Work out the finished part from the listing and answer in its coordinate system (mm). Face numbers are marked on the shaded views. A direction names the side the tool comes from. Coordinates: 2 decimals unless noted, no trailing zeros. Write each loop counter-clockwise with the first axis right and the second up, starting at its lowest first coordinate (ties: lowest second). Pieces come first, ordered by that corner, then holes. Notation, with made-up numbers: (-34.5, 5) - (-6.5, 5) arc R16 cw to (-6.5, 29) - close; hole circle Ø2 at (18, -18). An arc over 180 degrees is marked (long way). Answer as a JSON object with one key per item and string values. Group by question number.
from build123d import *

# Parameters (mm, degrees)
SKETCH1_W           = 60
SKETCH1_H           = 30
SKETCH1_R           = 2.3
BOSS_EXTRUDE1_DEPTH = 5
SKETCH3_W           = 5
SKETCH3_H           = 5
BOSS_EXTRUDE2_DEPTH = 35
SKETCH5_W           = 5
SKETCH5_H           = 5
SKETCH5_R           = 1.875
BOSS_EXTRUDE3_DEPTH = 2.5
SKETCH6_W           = 5
SKETCH6_H           = 30
BOSS_EXTRUDE4_DEPTH = 15
CUT_EXTRUDE1_REACH  = 64.048


with BuildPart() as part:
    # Sketch1 → Boss-Extrude1 (new body)
    with BuildSketch(Plane.XY):
        Rectangle(SKETCH1_W, SKETCH1_H)
        with Locations((-13.800714267, 9.000714267)):
            Circle(SKETCH1_R, mode=Mode.SUBTRACT)
        with Locations((5.999285733, 9.000714267)):
            Circle(SKETCH1_R, mode=Mode.SUBTRACT)
        with Locations((20, -5)):
            Circle(SKETCH1_R, mode=Mode.SUBTRACT)
    extrude(amount=BOSS_EXTRUDE1_DEPTH)

    # Sketch3 → Boss-Extrude2 (add)
    with BuildSketch(Plane.XY.offset(5)):
        with Locations((27.5, 12.5)):
            Rectangle(SKETCH3_W, SKETCH3_H)
        with Locations((-27.5, -12.5)):
            Rectangle(SKETCH3_W, SKETCH3_H)
    extrude(amount=BOSS_EXTRUDE2_DEPTH)

    # Sketch5 → Boss-Extrude3 (add)
    # profile 1 of 2: a face of its own
    with BuildSketch(Plane.XY.offset(40)):
        with Locations((-27.5, -7.5)):
            Rectangle(SKETCH5_W, SKETCH5_H)
        with Locations((-27.5, -7.5)):
            Circle(SKETCH5_R, mode=Mode.SUBTRACT)
    # profile 2 of 2: a face of its own
    with BuildSketch(Plane.XY.offset(40)):
        with Locations((27.5, 7.5)):
            Rectangle(SKETCH5_W, SKETCH5_H)
        with Locations((27.5, 7.5)):
            Circle(SKETCH5_R, mode=Mode.SUBTRACT)
    extrude(amount=-BOSS_EXTRUDE3_DEPTH)

    # Sketch6 → Boss-Extrude4 (add)
    with BuildSketch(Plane.ZY.offset(30)):
        with Locations((2.5, 0)):
            Rectangle(SKETCH6_W, SKETCH6_H)
    extrude(amount=BOSS_EXTRUDE4_DEPTH)

    # Sketch7 → Cut-Extrude1 (cut, up to next)
    with BuildSketch(Plane(origin=(0, 0, 0), x_dir=(-1, 0, 0), z_dir=(0, 0, -1)), mode=Mode.PRIVATE) as cut_extrude1_sk1:
        with BuildLine():
            Line((23.394171206, 9.42), (39.386735103, 9.42))
            ThreePointArc((39.386735103, 9.42), (43.815453154, -0.09), (39.386735103, -9.6))
            Line((39.386735103, -9.6), (23.394171206, -9.6))
            ThreePointArc((23.394171206, -9.6), (18.965453154, -0.09), (23.394171206, 9.42))
        make_face()
    cut_extrude1_tool1 = extrude(cut_extrude1_sk1.sketch, amount=-CUT_EXTRUDE1_REACH, mode=Mode.PRIVATE) & part.part
    add(cut_extrude1_tool1.solids().sort_by_distance((-31.390453, -0.09, 0))[0], mode=Mode.SUBTRACT)


solid = part.part
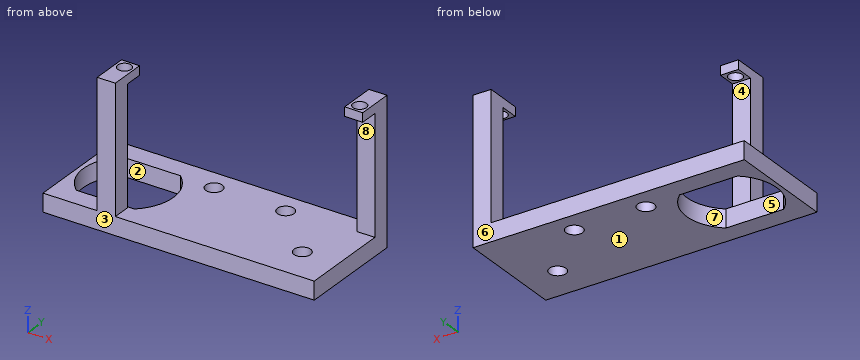
Q1. Section A-A on x = 20 is taken. Determine the outline of the cut face in (y, z), plus the area to 3 significant figures.
Q2. For a pull along Y with two mould halves and no side action, classify the marked faces 1, 2, 3 and 4 as +Y half, -Y half, draft (parallel to the pull), parting line (faces both ways), or undercut.
Q3. Flat-ended cylindrical pins translate along their axes: pin 1 Ø4 at (x, y) = (20, 10) entering from +Z; pin 2 Ø1 at (y, z) = (-10, 27) entering from +X; pin 3 Ø5.5 at (x, z) = (-28, 24.5) entering from +Y. Find the tip coordinate at first contact, or state that the pin passes through.
Q4. Consider L1, parallel to Y at x = 20, z = 1; L2, parallel to Y at x = 27.5, z = 38.9 (3 decimals); L3, parallel to Z at x = -16, y = -1.5. Determine where each line is inside the solid, lowest interval first. Write a range as from..to.
Q5. Section B-B on z = 20.5 is taken. Determine the outline of the cut face in (x, y).
Q6. Section C-C on x = -27 is taken. Determine the outline of the cut face in (y, z), plus the area to 3 significant figures.
Q7. Section D-D on y = 7.5 is taken. Determine the outline of the cut face in (x, z) (3 decimals), plus the area to 3 significant figures.
Q8. A tool of negligible diameter and unlimited length cuts with its end or side. For the marked faces 5, 6, 7 and 8, from which of +Z, -Z, +X, -X, +Y, -Y can it reach the whole face along a straight path? Write none if from no direction.
Numbers:
{
 "1": {"outline": "(-15, 0) - (-7.3, 0) - (-7.3, 5) - (-15, 5) - close; (-2.7, 0) - (15, 0) - (15, 5) - (-2.7, 5) - close", "area": "127 mm²"},
 "2": {"face 1": "draft", "face 2": "undercut", "face 3": "-Y half", "face 4": "+Y half"},
 "3": {"pin 1": "stops at z = 5", "pin 2": "stops at x = -25", "pin 3": "stops at y = -10"},
 "4": {"L1": "y = -15..-7.3, -2.7..15", "L2": "y = 5..5.625, 9.375..15", "L3": "z = 0..5"},
 "5": {"outline": "(-30, -15) - (-25, -15) - (-25, -10) - (-30, -10) - close; (25, 10) - (30, 10) - (30, 15) - (25, 15) - close"},
 "6": {"outline": "(-15, 0) - (-9.6, 0) - (-9.6, 5) - (-10, 5) - (-10, 37.5) - (-9.31, 37.5) - (-9.31, 40) - (-15, 40) - close; (-5.69, 37.5) - (-5, 37.5) - (-5, 40) - (-5.69, 40) - close; (9.42, 0) - (15, 0) - (15, 5) - (9.42, 5) - close", "area": "233 mm²"},
 "7": {"outline": "(-45, 0) - (-41.228, 0) - (-41.228, 5) - (-45, 5) - close; (-21.553, 0) - (-15.544, 0) - (-15.544, 5) - (-21.553, 5) - close; (-12.058, 0) - (4.256, 0) - (4.256, 5) - (-12.058, 5) - close; (7.742, 0) - (30, 0) - (30, 5) - (7.742, 5) - close; (25, 37.5) - (25.625, 37.5) - (25.625, 40) - (25, 40) - close; (29.375, 37.5) - (30, 37.5) - (30, 40) - (29.375, 40) - close", "area": "245 mm²"},
 "8": {"face 5": "-Z", "face 6": "+Z, -Z, +X, -X, +Y", "face 7": "+Z, -Z", "face 8": "+X, -X, -Y"}
}
